```python
from build123d import *

# Parameters (mm, degrees)
F4_W     = 14
F4_H     = 2
F5_DEPTH = 0.2
F6_R     = 0.6
F6_R_2   = 0.5
F7_DEPTH = 2


with BuildPart() as f3:
    # F3: sweep along a path in F0
    with BuildLine(Plane.XY) as f3_path:
        Line((0, -6.5), (2.1431406292, -4.6247519495))
        ThreePointArc((2.1431406292, -4.6247519495), (2.8247129707, -3.0442874784), (2.0261314134, -1.5195985601))
        Line((2.0261314134, -1.5195985601), (0.8, -0.6))
        ThreePointArc((0.8, -0.6), (0.211145618, 0.105572809), (0, 1))
        Line((0, 1), (0, 20))
        Line((0, 20), (1.1396454369, 23.6084911359))
        ThreePointArc((1.1396454369, 23.6084911359), (-0.1, 25.3), (-1.3396454369, 23.6084911359))
        Line((-1.3396454369, 23.6084911359), (-0.2, 20))
        Line((-0.2, 20), (-0.2, 0))
        Line((-0.2, 0), (-0.2, -5.5))
    # F2 (on plane+point) → F3 (sweep)
    with BuildSketch(Plane.XZ.offset(5.5)):
        with BuildLine():
            Line((-0.2, 0), (-0.2, 1))
            ThreePointArc((-0.2, 1), (-1.2, 0), (-0.2, -1))
            Line((-0.2, -1), (-0.2, 0))
        make_face()
    sweep(path=f3_path.line, transition=Transition.RIGHT)

    # F4 (on face) → F5 (join, through all)
    with BuildSketch(Plane.YZ.offset(-0.2)):
        with Locations((10.5, 0)):
            Rectangle(F4_W, F4_H)
    extrude(amount=F5_DEPTH)

    # F6 (on Top) → F7 (join)
    with BuildSketch(Plane.XY):
        with Locations((0, 15.5)):
            Circle(F6_R)
        with Locations((0, 5.5)):
            Circle(F6_R)
        with Locations((0, 26.2)):
            Circle(F6_R_2)
        with Locations((2.8, -3)):
            Circle(F6_R_2)
        with Locations((-0.7, -4.5)):
            Circle(F6_R_2)
        with Locations((0.75, -6.95)):
            Circle(F6_R_2)
    extrude(amount=F7_DEPTH)


solid = f3.part
```
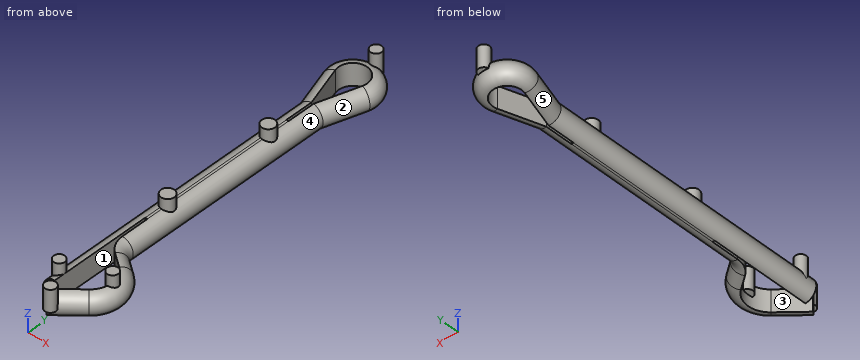
Could you check a few things on this model? Use its own coordinates, in mm. Face numbers are marked on the shaded views. A direction names the side the tool comes from. Coordinates: 2 decimals unless noted, no trailing zeros. Order: outer loops, then holes, each group sorted by start corner. A loop starts at its lowest first (then second) coordinate and runs counter-clockwise, first axis right, second up. Notation, with made-up numbers: M 70,-14 L 124,-14 A17 cw 124,0 Z; hole C 15,37.25 d7. An arc over 180 degrees is marked long. Use a Markdown table: item, result. Add a question column.
Q1. I want a section at B-B on y = 8.5. List the corners of the cut face in (x, z) for me.
Q2. Which directions (+Z, -Z, +X, -X, +Y, -Y) give clear straight access to the entire face, cutting with the end or side of a thin tool? Please do the marked faces 3, 4 and 5.
Q3. If I drill on L1, parallel to Y at x = 0.75, z = 1.35; L2, parallel to X at y = 24, z = 0.3; L3, parallel to Z at x = -1, y = 11.5, over which ranges is the centre line in solid material (lowest first)?
Q4. I'm going to push flat-ended pins straight in: pin 1 (1 mm diameter, centred on y = 18.5, z = 0.5, fed in from -X); pin 2 (1.6 mm diameter, centred on y = 18.5, z = -0.5, fed in from +X); pin 3 (1 mm diameter, centred on x = 2, z = 1, fed in from -Y); pin 4 (3 mm diameter, centred on x = 0.5, y = 0, fed in from -Z). Where does each tip first touch, or does it pass through?
Q5. We'd pull the mould along Y, two halves only. Please class the marked faces 1 and 2: pulls with the +Y half, pulls with the -Y half, needs draft (parallel to the pull), parting line crosses it, or undercut.
Checked values:
| question | item | result |
|---|---|---|
| 1 | outline | M -0.2,-1 L 0,-1 A1 ccw 0,1 L -0.2,1 A1 ccw Z |
| 2 | face 3 | +Z, -Z |
| 2 | face 4 | +X |
| 2 | face 5 | -X |
| 3 | L1 | -7.45 to -6.45 |
| 3 | L2 | -2.35 to -1.4, 1.2 to 2.15 |
| 3 | L3 | -0.6 to 0.6 |
| 4 | pin 1 | x = -1.2 |
| 4 | pin 2 | x = 1 |
| 4 | pin 3 | y = -6.08 |
| 4 | pin 4 | z = -1 |
| 5 | face 1 | needs draft |
| 5 | face 2 | undercut |
